Can you work these out from the model? Positions are in its coordinate system, mm. Face numbers are marked on the shaded views. Give positions to 0.01 mm unless a question says otherwise; leave off trailing zeros. Order: outer loops, then holes, each group sorted by start corner. A loop starts at its lowest first (then second) coordinate and runs counter-clockwise, first axis right, second up. Notation, with made-up numbers: (5.5, 19.5) - (30.5, 19.5) arc R26 ccw to (30.5, 53.5) - close; hole circle Ø8 at (-0.5, 30). An arc over 180 degrees is marked (long way). One line per question, with ' | ' between items.
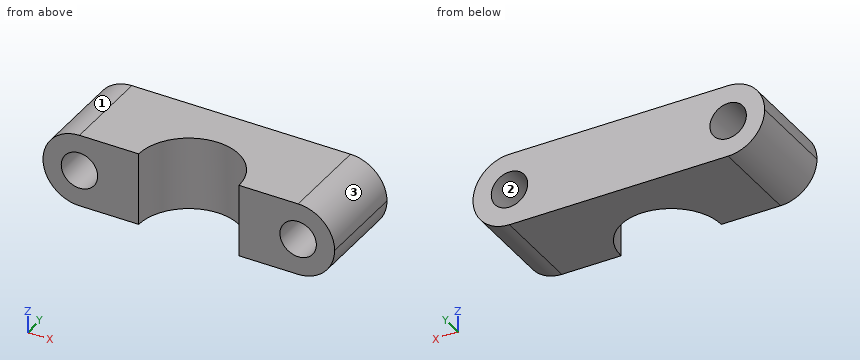
```python
from build123d import *

# Parameters (mm, degrees)
BOSS_EXTRUDE1_DEPTH = 6.35
SKETCH2_R           = 3.175
CUT_EXTRUDE1_DEPTH  = 31.618591166
FILLET1_R           = 6.35


with BuildPart() as part:
    # Sketch1 → Boss-Extrude1 (new, symmetric)
    with BuildSketch(Plane.XY):
        with BuildLine():
            Line((-8.73125, 0), (-25.4, 0))
            Line((-25.4, 0), (-25.4, 15.875))
            Line((-25.4, 15.875), (25.4, 15.875))
            Line((25.4, 15.875), (25.4, 0))
            Line((25.4, 0), (8.73125, 0))
            ThreePointArc((8.73125, 0), (0, 8.73125), (-8.73125, 0))
        make_face()
    extrude(amount=BOSS_EXTRUDE1_DEPTH, both=True)

    # Sketch2 → Cut-Extrude1 (cut, through all)
    with BuildSketch(Plane(origin=(0, 0, 0), x_dir=(1, 0, 0), z_dir=(0, 1, 0))):
        with Locations(Location((-19.05, 0, 0), (0, 0, 270))):
            Circle(SKETCH2_R)
        with Locations(Location((19.05, 0, 0), (0, 0, 270))):
            Circle(SKETCH2_R)
    extrude(amount=CUT_EXTRUDE1_DEPTH, mode=Mode.SUBTRACT)

    # Fillet1
    fillet1_edges = [part.edges().sort_by_distance(p)[0] for p in [
        (25.4, 7.9375, -6.35),
        (25.4, 7.9375, 6.35),
        (-25.4, 7.9375, -6.35),
        (-25.4, 7.9375, 6.35),
    ]]
    fillet(fillet1_edges, radius=FILLET1_R - 0.0001)  # a hair under: the kernel refuses the full size


solid = part.part
```
(1) Imagine slicing it at B-B (z = -2.25). List the corners of the cut face in (x, y) for me (1 decimal).
Answer below:
outline: (-25, 0) - (-21.3, 0) - (-21.3, 15.9) - (-25, 15.9) - close; (-16.8, 0) - (-8.7, 0) arc R8.7 cw to (8.7, 0) - (16.8, 0) - (16.8, 15.9) - (-16.8, 15.9) - close; (21.3, 0) - (25, 0) - (25, 15.9) - (21.3, 15.9) - close
(2) Imagine slicing it at D-D (x = 0). List the corners of the cut face in (y, z) for me (3 decimals).
Answer below:
outline: (8.731, -6.35) - (15.875, -6.35) - (15.875, 6.35) - (8.731, 6.35) - close
(3) Will these pins go through, and if not, where does the flat tip stop? pin 1 (1 mm diameter, centred on y = 14, z = -5, fed in from +X); pin 2 (5 mm diameter, centred on y = 12, z = 3, fed in from -X); pin 3 (5 mm diameter, centred on x = -19.05, z = 0, fed in from -Y).
Answer below:
pin 1: x = 23.53 | pin 2: x = -25.38 | pin 3: through
(4) If I drill on line 1 (X direction, y = 9.5, z = 0) (3 decimals); line 2 (Z direction, x = -19.05, y = 4) (3 decimals); line 3 (X direction, y = 3, z = 0) (3 decimals), over which ranges is the centre line in solid material (lowest first)?
Answer below:
line 1: -25.4 to -22.225, -15.875 to 15.875, 22.225 to 25.4 | line 2: -6.35 to -3.175, 3.175 to 6.35 | line 3: -25.4 to -22.225, -15.875 to -8.2, 8.2 to 15.875, 22.225 to 25.4
(5) If we mould it in two halves opening along X, with no side actions, what happens to the marked faces 1, 2 and 3? For each: released by +X, released by -X, zero draft, split by the parting line, or undercut.
Answer below:
face 1: released by -X | face 2: undercut | face 3: released by +X
(6) Imagine slicing it at A-A (y = 7). Count the separate pieces of the cut face and the enclosed holes in it, and give its area (3 significant figures).
Answer below:
separate pieces: 2 | enclosed holes: 2 | area: 415 mm^2
